Model file for the job. Use its own axes, mm. A direction names the side the tool comes from. Round coordinates to 2 decimals unless told otherwise and drop trailing zeros. Answer in a Markdown table with one row per item.
from build123d import *

# Parameters (mm, degrees)
F1_R     = 12.5
F3_DEPTH = 10
F4_SIZE2 = 1.4106158457
F4_SIZE  = 8
F2_R     = 5
F6_R     = 5.5
F7_DEPTH = 17
F8_SIZE  = 1


with BuildPart() as f3:
    # F1 (on offset) → F3 (new body)
    with BuildSketch(Plane.XY.offset(-22.5)):
        Circle(F1_R)
    extrude(amount=F3_DEPTH)

    # F4
    f4_edges = [f3.edges().sort_by_distance(p)[0] for p in [
        (-12.5, 0, -12.5),
    ]]
    f4_side = f3.faces().sort_by_distance((0, 0, -12.5))[0]
    chamfer(f4_edges, length=F4_SIZE, length2=F4_SIZE2, reference=f4_side)

    # F2 (on Top) → F5 (revolve)
    with BuildSketch(Plane.XY):
        with Locations((17.5, 0)):
            Circle(F2_R)
    revolve(axis=Axis((0, 2.5942958891, 0), (0, -1, 0)))

    # F6 (on face) → F7 (join)
    with BuildSketch(Plane(origin=(0, 0, -22.5), x_dir=(1, 0, 0), z_dir=(0, 0, -1))):
        Circle(F6_R)
    extrude(amount=F7_DEPTH)

    # F8
    f8_edges = [f3.edges().sort_by_distance(p)[0] for p in [
        (-5.5, 0, -39.5),
    ]]
    chamfer(f8_edges, length=F8_SIZE)


solid = f3.part
1. Wall check: probe 1 along Y at (x, z) = (12.5, 12); probe 2 along X at (y, z) = (4.25, -4); probe 3 along X at (y, z) = (1, -2). Give the ranges that are in metal, low to high.
Verdict:
| item | result |
|---|---|
| probe 1 | y = -5 to 5 |
| probe 2 | x = -19.73 to -14.32, 14.32 to 19.73 |
| probe 3 | x = -22.31 to -12.44, 12.44 to 22.31 |
2. Tool access for faces 1 (the flat face through (3, -5, -22.5)), 2 (the flat face through (0, 0, -39.5)), 3 (the flat face through (0, -2, -12.5)), 4 (the conical face through (0.12, 7.67, -13.06)): list every direction of +Z, -Z, +X, -X, +Y, -Y with a clear straight run to the whole face (end or side of a thin tool).
Verdict:
| item | result |
|---|---|
| face 1 | -Z |
| face 2 | -Z, +X, -X, +Y, -Y |
| face 3 | -Y |
| face 4 | +Y |
3. Mould opens along Z. For faces 5 (the conical face through (-4, 3, -39)), 6 (the flat face through (0, 2, -12.5)), 7 (the cylindrical face through (-1.19, 5.37, -30.39)) say: +Z half, -Z half, draft (parallel to the pull), parting line (faces both ways), or undercut.
Verdict:
| item | result |
|---|---|
| face 5 | -Z half |
| face 6 | undercut |
| face 7 | draft |
4. Pin check, flat tips, straight feed: pin 1 (4 mm diameter, centred on x = -4.5, z = -33, fed in from -Y); pin 2 (5 mm diameter, centred on x = -2, y = -2, fed in from +Z); pin 3 (12 mm diameter, centred on x = 3, z = -1, fed in from +Y); pin 4 (5 mm diameter, centred on x = 5.5, y = 1, fed in from +Z). Stop position of each tip, or through.
Verdict:
| item | result |
|---|---|
| pin 1 | stops at y = -4.9 |
| pin 2 | stops at z = 22.5 |
| pin 3 | passes through |
| pin 4 | stops at z = 22.28 |
